```python
from build123d import *

# Parameters (mm, degrees)
F1_DEPTH = 16
F2_DEPTH = 4.5
F3_R     = 13.5
F3_R_2   = 6
F4_DEPTH = 7.5


with BuildPart() as f1:
    # F0 (on Top) → F1 (new body)
    with BuildSketch(Plane.XY):
        with BuildLine():
            Line((4, 0), (13.5, 0))
            ThreePointArc((13.5, 0), (11.4985218419, 7.0734712448), (6.0875562295, 12.0495501639))
            ThreePointArc((6.0875562295, 12.0495501639), (0, 13.5), (-6.0875562295, 12.0495501639))
            ThreePointArc((-6.0875562295, 12.0495501639), (-11.4985218419, 7.0734712448), (-13.5, 0))
            Line((-13.5, 0), (-4, 0))
            ThreePointArc((-4, 0), (0, 4), (4, 0))
        make_face()
        with BuildLine():
            ThreePointArc((6.0875562295, -12.0495501639), (11.4985218419, -7.0734712448), (13.5, 0))
            Line((13.5, 0), (4, 0))
            ThreePointArc((4, 0), (0, -4), (-4, 0))
            Line((-4, 0), (-13.5, 0))
            ThreePointArc((-13.5, 0), (-11.4985218419, -7.0734712448), (-6.0875562295, -12.0495501639))
            ThreePointArc((-6.0875562295, -12.0495501639), (0, -13.5), (6.0875562295, -12.0495501639))
        make_face()
    extrude(amount=F1_DEPTH)

    # F0 (on Top) → F2 (join)
    with BuildSketch(Plane.XY):
        with BuildLine():
            ThreePointArc((-13.5, 0), (-11.4985218419, 7.0734712448), (-6.0875562295, 12.0495501639))
            Line((-6.0875562295, 12.0495501639), (-24, 3))
            Line((-24, 3), (-24, 0))
            Line((-24, 0), (-21.25, 0))
            ThreePointArc((-21.25, 0), (-18.5, 2.75), (-15.75, 0))
            Line((-15.75, 0), (-13.5, 0))
        make_face()
        with BuildLine():
            Line((-24, -3), (-6.0875562295, -12.0495501639))
            ThreePointArc((-6.0875562295, -12.0495501639), (-11.4985218419, -7.0734712448), (-13.5, 0))
            Line((-13.5, 0), (-15.75, 0))
            ThreePointArc((-15.75, 0), (-18.5, -2.75), (-21.25, 0))
            Line((-21.25, 0), (-24, 0))
            Line((-24, 0), (-24, -3))
        make_face()
        with BuildLine():
            ThreePointArc((6.0875562295, 12.0495501639), (11.4985218419, 7.0734712448), (13.5, 0))
            Line((13.5, 0), (15.75, 0))
            ThreePointArc((15.75, 0), (18.5, 2.75), (21.25, 0))
            Line((21.25, 0), (24, 0))
            Line((24, 0), (24, 3))
            Line((24, 3), (6.0875562295, 12.0495501639))
        make_face()
        with BuildLine():
            Line((15.75, 0), (13.5, 0))
            ThreePointArc((13.5, 0), (11.4985218419, -7.0734712448), (6.0875562295, -12.0495501639))
            Line((6.0875562295, -12.0495501639), (24, -3))
            Line((24, -3), (24, 0))
            Line((24, 0), (21.25, 0))
            ThreePointArc((21.25, 0), (18.5, -2.75), (15.75, 0))
        make_face()
    extrude(amount=F2_DEPTH)

    # F3 (on face) → F4 (cut)
    with BuildSketch(Plane.XY.offset(16)):
        Circle(F3_R)
        Circle(F3_R_2, mode=Mode.SUBTRACT)
    extrude(amount=-F4_DEPTH, mode=Mode.SUBTRACT)


solid = f1.part
```
CAD build for the part. Positions are in the model's coordinates, mm. A direction names the side the tool comes from. Coordinates: 2 decimals unless noted, no trailing zeros. Order: outer loops, then holes, each group sorted by start corner. A loop starts at its lowest first (then second) coordinate and runs counter-clockwise, first axis right, second up. Notation, with made-up numbers: M 21,13 L 35,13 A30 ccw 35,43 Z; hole C 86.25,44.5 d7. An arc over 180 degrees is marked long. Answer as CSV lines item,"result".
1) Cut at B-B (z = 1.5). List the corners of the cut face in (x, y).
Verdict:
outline,"M -24,-3 L -6.09,-12.05 A13.5 ccw 6.09,-12.05 L 24,-3 L 24,3 L 6.09,12.05 A13.5 ccw -6.09,12.05 L -24,3 Z; hole C -18.5,0 d5.5; hole C 0,0 d8; hole C 18.5,0 d5.5"
2) 3-axis set-ups, long thin cutter, end or side, ignore diameter. For faces 5 (the flat face through (15.17, 7.46, 2.22)), 6 (the cylindrical face through (-6, 0, 12)): which of +Z, -Z, +X, -X, +Y, -Y reach the whole face in a straight line?
Verdict:
face 5,"+Z, -Z, +X, +Y"
face 6,"+Z"
3) Cut at A-A (x = 0). List the corners of the cut face in (y, z), then the cut area to 4 significant figures.
Verdict:
outline,"M -13.5,0 L -4,0 L -4,16 L -6,16 L -6,8.5 L -13.5,8.5 Z; M 4,0 L 13.5,0 L 13.5,8.5 L 6,8.5 L 6,16 L 4,16 Z"
area,"191.5 mm2"
4) Cut at D-D (z = 12). List the corners of the cut face in (x, y), then the cut area to 3 significant figures.
Verdict:
outline,"C 0,0 d12; hole C 0,0 d8"
area,"62.8 mm2"
5) Drill centre lines: L1, parallel to Y at x = 0, z = 7.5; L2, parallel to Y at x = 0, z = 11.5; L3, parallel to Z at x = -6, y = 7.5. Where is each one in solid material? Low to high. Write a range as from..to.
Verdict:
L1,"-13.5..-4, 4..13.5"
L2,"-6..-4, 4..6"
L3,"0..8.5"
6) Flat gauge pins, fed straight in: P1, Ø5, axis at x = -13, z = 10, coming from the -Y side; P2, Ø8, axis at y = 4.5, z = 10.5, coming from the -X side; P3, Ø6.5, axis at x = 18.5, y = 0, coming from the +Z side. Where does each tip first touch, or does it go through?
Verdict:
P1,"y = -7.83"
P2,"x = -13.46"
P3,"z = 4.5"
7) Mould opens along X. For faces 1 (the flat face through (-14.918, 7.588, 2.218)), 2 (the flat face through (14.918, -7.588, 2.218)), 3 (the flat face through (-1.42, -3.92, 16)), 4 (the cylindrical face through (16.318, 1.673, 2.218)) say: released by +X, released by -X, zero draft, split by the parting line, or undercut.
Verdict:
face 1,"released by -X"
face 2,"released by +X"
face 3,"zero draft"
face 4,"undercut"
8) Cut at C-C (y = 1.25). List the corners of the cut face in (x, z).
Verdict:
outline,"M -24,0 L -20.95,0 L -20.95,4.5 L -24,4.5 Z; M -16.05,0 L -3.8,0 L -3.8,16 L -5.87,16 L -5.87,8.5 L -13.44,8.5 L -13.44,4.5 L -16.05,4.5 Z; M 3.8,0 L 16.05,0 L 16.05,4.5 L 13.44,4.5 L 13.44,8.5 L 5.87,8.5 L 5.87,16 L 3.8,16 Z; M 20.95,0 L 24,0 L 24,4.5 L 20.95,4.5 Z"
